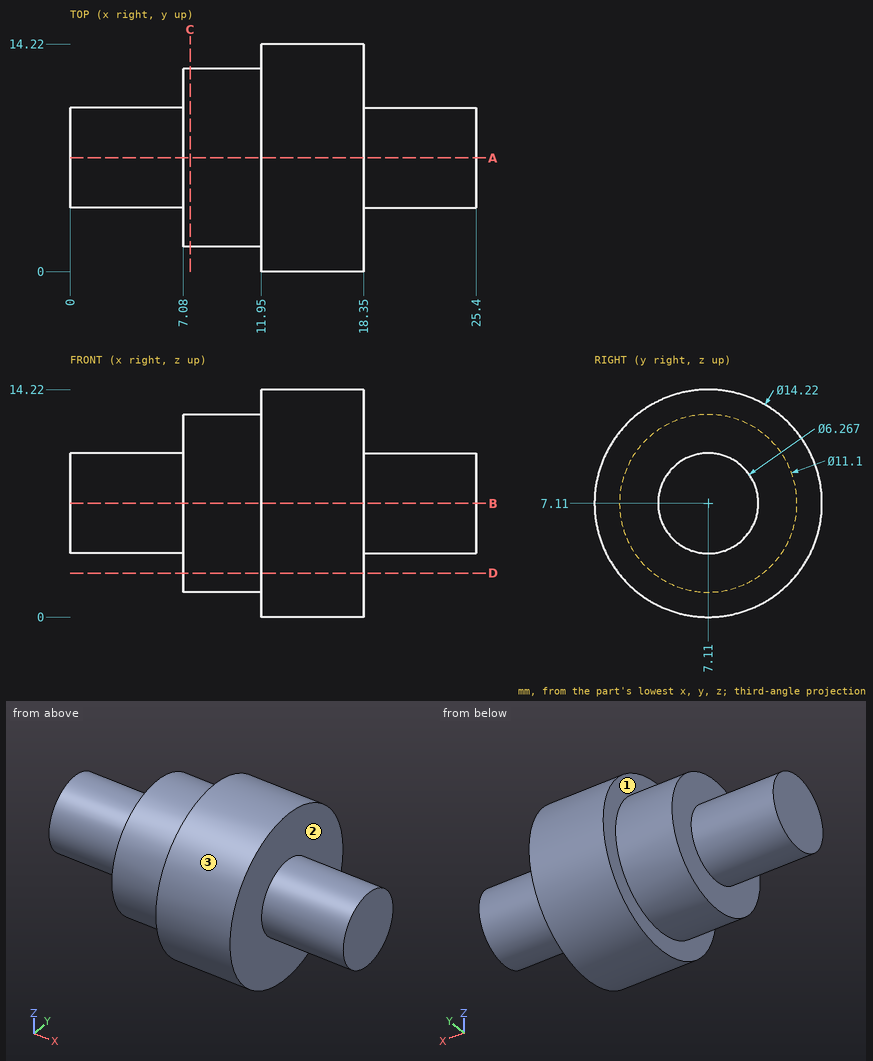
Geometry check sheet. Reference: drawing and pictorial views, mm from the part's lowest x, y, z. A direction names the side the tool comes from. Give positions to 0.01 mm unless a question says otherwise; leave off trailing zeros. Loops run counter-clockwise (first coordinate to the right, second up) from the corner with the lowest first, then second, coordinate; pieces in that order, holes last. Notation, with made-up numbers: (3, -5.75) -> (15, -5.75) arc R32 cw to (15, 33.25) -> close; hole circle Ø10 at (80.5, 45). An arc over 180 degrees is marked (long way). Answer in a Markdown table with one row per item. Add a question column.
1) Cross-section at A-A on y = 7.11. Record the boundary of the cut face in (x, z), and give its area (3 significant figures).
2) Set-up check for the marked faces 1, 2 and 3: record each of +Z, -Z, +X, -X, +Y, -Y from which the full face is reachable in a straight line by a thin tool's end or side.
3) Material ranges on probe 1 along X at (y, z) = (10.75, 10); probe 2 along X at (y, z) = (12.5, 2.75); probe 3 along Z at (x, y) = (4, 7), recorded low to high. Write a range as from..to.
4) Cross-section at D-D on z = 2.75. Record the boundary of the cut face in (x, y).
5) Cross-section at C-C on x = 7.5. Record the boundary of the cut face in (y, z).
6) Gauge pin test, flat ends, axial feed: P1, Ø5, axis at y = 2, z = 3, coming from the +X side; P2, Ø4, axis at x = 22, z = 5, coming from the +Y side; P3, Ø5, axis at x = 5.5, y = 4.5, coming from the -Z side. Record the tip position at first contact, or that the pin passes through.
Outcome:
| question | item | result |
|---|---|---|
| 1 | outline | (0, 3.98) -> (7.08, 3.98) -> (7.08, 1.56) -> (11.95, 1.56) -> (11.95, 0) -> (18.35, 0) -> (18.35, 3.98) -> (25.4, 3.98) -> (25.4, 10.24) -> (18.35, 10.24) -> (18.35, 14.22) -> (11.95, 14.22) -> (11.95, 12.66) -> (7.08, 12.66) -> (7.08, 10.24) -> (0, 10.24) -> close |
| 1 | area | 234 mm^2 |
| 2 | face 1 | -X |
| 2 | face 2 | +X |
| 2 | face 3 | +X, -X |
| 3 | probe 1 | x = 7.08..18.35 |
| 3 | probe 2 | x = 11.95..18.35 |
| 3 | probe 3 | z = 3.98..10.24 |
| 4 | outline | (7.08, 3.68) -> (11.95, 3.68) -> (11.95, 1.49) -> (18.35, 1.49) -> (18.35, 12.73) -> (11.95, 12.73) -> (11.95, 10.54) -> (7.08, 10.54) -> close |
| 5 | outline | circle Ø11.1 at (7.11, 7.11) |
| 6 | P1 | stops at x = 18.35 |
| 6 | P2 | stops at y = 10.24 |
| 6 | P3 | stops at z = 1.6 |
